Here's how the part is built. I have some questions about the finished solid (model axes, mm). Round coordinates to 2 decimals unless told otherwise and drop trailing zeros. Loops run counter-clockwise (first coordinate to the right, second up) from the corner with the lowest first, then second, coordinate; pieces in that order, holes last. Notation, with made-up numbers: M 86.25,13.5 L 120.25,13.5 A32 cw 120.25,51.5 Z; hole C 74.5,10.25 d11. An arc over 180 degrees is marked long. Answer as a JSON object with one key per item and string values.
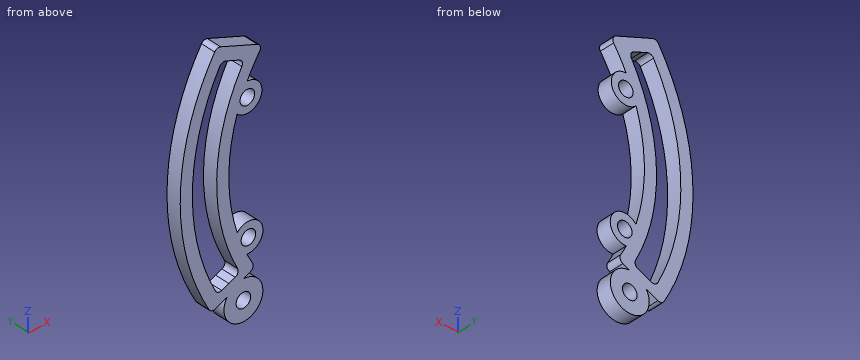
Autodesk Inventor part; units mm, degrees
ref_plane "YZ Plane" through (0, 0, 0) normal (1, 0, 0) x (0, 1, 0)
ref_plane "XZ Plane" through (0, 0, 0) normal (0, 1, 0) x (-1, 0, 0)
ref_plane "XY Plane" through (0, 0, 0) normal (0, 0, 1) x (1, 0, 0)
sketch "Sketch1" plane through (0, 0, 0) normal (0, 1, 0) x (-1, 0, 0)
  circle A0 centre (32.4474, 13.089) radius 1.5
  circle A1 centre (32.2267, -13) radius 1.5
  arc A2 (39.8573, -23.4618) -> (38.7049, 25.3179) centre (0, 0) ccw
  line L0 (32.9955, 20.319) -> (35.5948, 21.3676)
  line L1 (29.1983, 21.483) -> (38.7049, 25.3179)
  circle A3 centre (33.2491, -24.1954) radius 1.5
  line L2 (36.25, -19.685) -> (38.5713, -20.6475)
  line L3 (35.5948, 21.3676) -> (37.6913, 22.2133)
  line L4 (33.9272, -18.7219) -> (36.25, -19.685)
  arc A4 (33.9272, -18.7219) -> (32.9955, 20.319) centre (0, 0) ccw
  arc A5 (38.5713, -20.6475) -> (37.6913, 22.2133) centre (0, 0) ccw
  arc A6 (32.4841, 16.0888) -> (29.1983, 21.483) centre (0, 0) ccw
  arc A7 (30.7875, -19.1361) -> (32.5357, -15.984) centre (0, 0) ccw
  arc A8 (34.5198, -11.0656) -> (34.5553, 10.9543) centre (0, 0) ccw
  arc A9 (32.4841, 16.0888) -> (34.5553, 10.9543) centre (32.4474, 13.089) ccw
  arc A10 (34.5198, -11.0656) -> (32.5357, -15.984) centre (32.2267, -13) ccw
  line L5 (33.2491, -20.1954) -> (30.7875, -19.1361)
  line L6 (36.643, -22.0786) -> (39.8573, -23.4618)
  arc A11 (33.2491, -20.1954) -> (36.643, -22.0786) centre (33.2491, -24.1954) ccw
  dimension "d29" = 4
  dimension "d30" = 3
  dimension "d31" = 3
  dimension "d32" = 46.25
  dimension "d33" = 43.75
  dimension "d34" = 38.75
  dimension "d35" = 36.25
  dimension "d36" = 36.25
  dimension "d37" = 0.764
  dimension "d38" = 45.253
  dimension "d39" = 0.764
  dimension "d40" = 0.3882
  dimension "d41" = 2.5
  dimension "d42" = 2.1071
  dimension "d43" = 43.1688
  dimension "d44" = 44.3514
  dimension "d45" = 2.0605
  dimension "d46" = 2.0432
  dimension "d47" = 39.4934
  dimension "d48" = 29.5173
  dimension "d49" = 9.2767
  dimension "d50" = 1.6208
  dimension "d51" = 33.4149
  dimension "d52" = 5.7959
  dimension "d53" = 4.2998
  dimension "d54" = 26.089
extrude "Extrusion1" add sketch "Sketch1" along normal blind 3
fillet "Fillet1" radius 1 8 edges at (-29.1983, 1.5, 21.483) (-38.7049, 1.5, 25.3179) (-38.5713, 1.5, -20.6475) (-30.7875, 1.5, -19.1361) (-33.9272, 1.5, -18.7219) (-39.8573, 1.5, -23.4618) (-32.9955, 1.5, 20.319) (-37.6913, 1.5, 22.2133)
properties part number "reverse gear reverse gear"
Item 1: For P1, Ø1.5, axis at x = -32, y = 1.5, coming from the +Z side, with a flat end and sliding along its axis, tell me the tip position at first contact or that it passes through.
Solution:
{"P1": "stops at z = 22.92"}
Item 2: I want a section at D-D on z = -13. List the corners of the cut face in (x, y) for me.
Solution:
{"outline": "M -44.39,0 L -41.77,0 L -41.77,3 L -44.39,3 Z; M -36.5,0 L -33.73,0 L -33.73,3 L -36.5,3 Z; M -30.73,0 L -29.23,0 L -29.23,3 L -30.73,3 Z"}
Item 3: If I drill on L1, parallel to Z at x = -34, y = 2; L2, parallel to X at y = 2.5, z = 18; L3, parallel to X at y = 2.7, z = -20, over which ranges is the centre line in solid material (lowest first)? Write a range as from..to.
Solution:
{"L1": "z = -28.12..-25.49, -22.9..-10.58, 10.52..18.59, 20.72..23.42", "L2": "x = -42.6..-39.88, -34.32..-31.47", "L3": "x = -41.7..-38.89, -37.01..-32.8"}
Item 4: I want a section at B-B on x = -43.25. List the corners of the cut face in (y, z) for me, plus the area to 3 significant figures.
Solution:
{"outline": "M 0,-16.39 L 3,-16.39 L 3,-6.6 L 0,-6.6 Z; M 0,6.6 L 3,6.6 L 3,16.39 L 0,16.39 Z", "area": "58.7 mm2"}
Item 5: I want a section at C-C on y = 1.05. Count the separate pieces of the cut face and the enclosed holes in it, plus the area to 3 significant figures.
Solution:
{"separate pieces": "1", "enclosed holes": "4", "area": "330 mm2"}
Item 6: I want a section at A-A on z = -7. List the corners of the cut face in (x, y) for me.
Solution:
{"outline": "M -45.72,0 L -43.19,0 L -43.19,3 L -45.72,3 Z; M -38.11,0 L -35.57,0 L -35.57,3 L -38.11,3 Z"}
